Autodesk Inventor part; units mm, degrees
ref_plane "YZ Plane" through (0, 0, 0) normal (1, 0, 0) x (0, 1, 0)
ref_plane "XZ Plane" through (0, 0, 0) normal (0, 1, 0) x (-1, 0, 0)
ref_plane "XY Plane" through (0, 0, 0) normal (0, 0, 1) x (1, 0, 0)
sketch "Sketch1" plane through (0, 0, 0) normal (0, 0, 1) x (1, 0, 0)
  circle A0 centre (0, 0) radius 76.2
  dimension "d0" = 152.4
extrude "Extrusion1" add sketch "Sketch1" along normal blind 38.1
sketch "Sketch2" plane through (0, 0, 38.1) normal (0, 0, 1) x (1, 0, 0)
  circle A0 centre (0, 0) radius 6.35
  dimension "d3" = 12.7
extrude "Extrusion2" cut sketch "Sketch2" against normal blind 38.1
sketch "Sketch3" plane through (0, 0, 38.1) normal (0, 0, 1) x (1, 0, 0)
  point P0 (0, 0)
fillet "Fillet1" radius 5.08 2 edges at (-76.2, 0, 38.1) (-76.2, 0, 0)
properties part number "6 inch wheel"
Design review of the part built by this model. Coordinates are the model's own, in mm. Give positions to 0.01 mm unless a question says otherwise; leave off trailing zeros. Order: outer loops, then holes, each group sorted by start corner. A loop starts at its lowest first (then second) coordinate and runs counter-clockwise, first axis right, second up.
1. To check wall thickness, follow L1, parallel to Y at x = 0, z = 29; L2, parallel to Y at x = -68.5, z = 17; L3, parallel to X at y = -53, z = 19. State the ranges of each line that lie inside material, in increasing order.
Solution:
L1: y = -76.2 to -6.35, 6.35 to 76.2
L2: y = -33.38 to 33.38
L3: x = -54.75 to 54.75
2. For pin 1 Ø4 at (y, z) = (-19.5, 30) entering from -X; pin 2 Ø10 at (x, z) = (-25.5, 9) entering from +Y; pin 3 Ø7.5 at (x, y) = (0, 0) entering from +Z; pin 4 Ø2 at (x, z) = (8.5, 4.5) entering from +Y, all flat-tipped, find the tip position at first contact; note any pin that passes through.
Solution:
pin 1: stops at x = -74.16
pin 2: stops at y = 73.39
pin 3: passes through
pin 4: stops at y = 75.82
3. Add section C-C, the plane z = 30.5. State the section outline as (x, y) points, then the cut area to 3 significant figures.
Solution:
outline: circle Ø152.4 at (0, 0); hole circle Ø12.7 at (0, 0)
area: 18,100 mm2
4. Mouldability with a two-part tool opening along X and no side actions: class faces 1 (the cylindrical face through (-60.47, 46.367, 18.854)), 2 (the flat face through (-1, -15, 38.1)), 3 (the cylindrical face through (-1.38, -6.2, 19.32)) as +X half, -X half, draft (parallel to the pull), parting line (faces both ways), or undercut.
Solution:
face 1: parting line
face 2: draft
face 3: undercut
5. Add section A-A, the plane x = 0. State the section outline as (y, z) points.
Solution:
outline: (-76.2, 5.08) arc R5.08 ccw to (-71.12, 0) - (-6.35, 0) - (-6.35, 38.1) - (-71.12, 38.1) arc R5.08 ccw to (-76.2, 33.02) - close; (6.35, 0) - (71.12, 0) arc R5.08 ccw to (76.2, 5.08) - (76.2, 33.02) arc R5.08 ccw to (71.12, 38.1) - (6.35, 38.1) - close
